Drawing for the job (mm, zero at the part's lowest x, y, z). A direction names the side the tool comes from. Give positions to 0.01 mm unless a question says otherwise; leave off trailing zeros. Loops run counter-clockwise (first coordinate to the right, second up) from the corner with the lowest first, then second, coordinate; pieces in that order, holes last. Notation, with made-up numbers: (89, 49) -> (96, 49) arc R17 cw to (96, 70) -> close; hole circle Ø9 at (65.5, -21.5). An arc over 180 degrees is marked (long way). Answer in a Markdown table with one row per item. Add a question column.
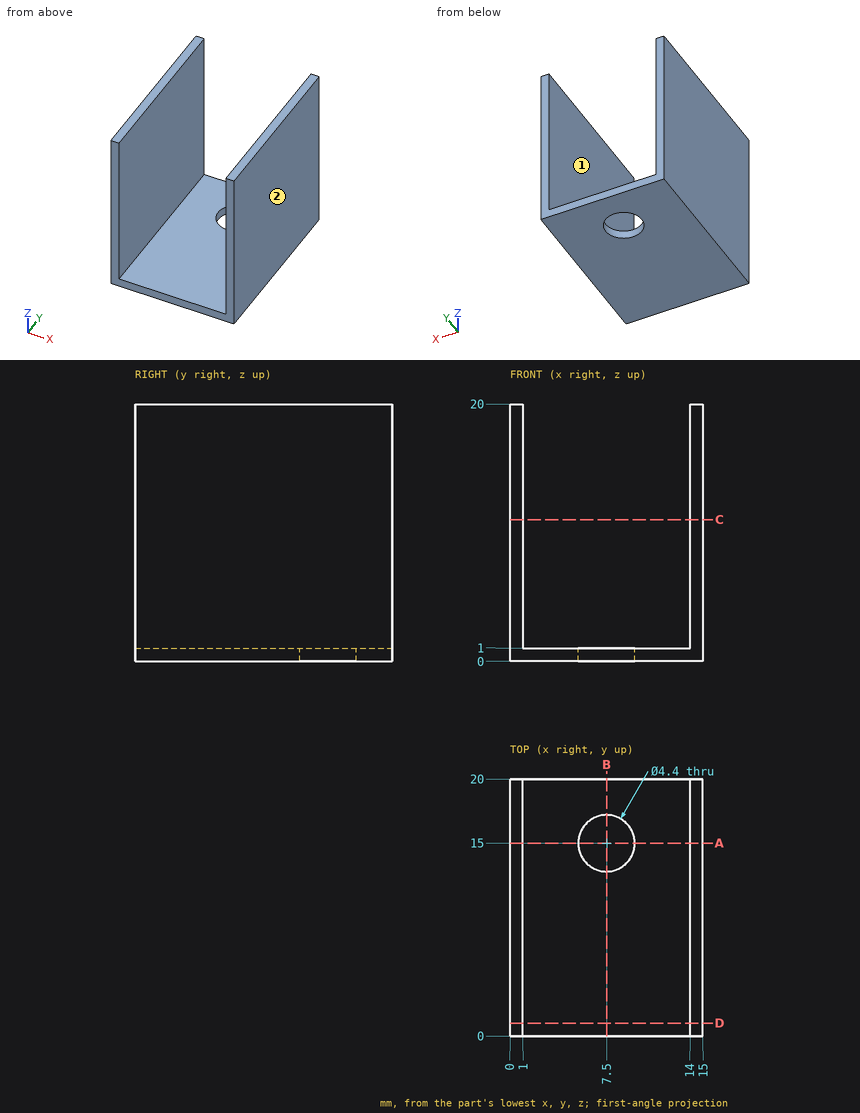
(1) Saw through at B-B, the plane x = 7.5. List the corners of the cut face in (y, z), then the cut area to 3 significant figures.
(2) Wall check: line 1 along X through (y, z) = (18, 8); line 2 along Y through (x, z) = (7.5, 0.7); line 3 along Z through (x, y) = (3.5, 11.5). Give the ranges that are in metal, low to high. Write a range as from..to.
(3) Saw through at D-D, the plane y = 1. List the corners of the cut face in (x, z).
(4) 3-axis set-ups, long thin cutter, end or side, ignore diameter. For the marked faces 1 and 2: which of +Z, -Z, +X, -X, +Y, -Y reach the whole face in a straight line?
(5) Saw through at C-C, the plane z = 11. List the corners of the cut face in (x, y), then the cut area to 3 significant figures.
(6) Saw through at A-A, the plane y = 15. List the corners of the cut face in (x, z), then the cut area to 3 significant figures.
(7) Flat gauge pin, fed straight in: pin 1 Ø3 at (x, y) = (4, 7.5) entering from +Z. Where does the tip first touch, or does it go through?
Worked answers:
| question | item | result |
|---|---|---|
| 1 | outline | (0, 0) -> (12.8, 0) -> (12.8, 1) -> (0, 1) -> close; (17.2, 0) -> (20, 0) -> (20, 1) -> (17.2, 1) -> close |
| 1 | area | 15.6 mm^2 |
| 2 | line 1 | 0..1, 14..15 |
| 2 | line 2 | 0..12.8, 17.2..20 |
| 2 | line 3 | 0..1 |
| 3 | outline | (0, 0) -> (15, 0) -> (15, 20) -> (14, 20) -> (14, 1) -> (1, 1) -> (1, 20) -> (0, 20) -> close |
| 4 | face 1 | +Z, +Y, -Y |
| 4 | face 2 | +Z, -Z, +X, +Y, -Y |
| 5 | outline | (0, 0) -> (1, 0) -> (1, 20) -> (0, 20) -> close; (14, 0) -> (15, 0) -> (15, 20) -> (14, 20) -> close |
| 5 | area | 40.0 mm^2 |
| 6 | outline | (0, 0) -> (5.3, 0) -> (5.3, 1) -> (1, 1) -> (1, 20) -> (0, 20) -> close; (9.7, 0) -> (15, 0) -> (15, 20) -> (14, 20) -> (14, 1) -> (9.7, 1) -> close |
| 6 | area | 48.6 mm^2 |
| 7 | pin 1 | z = 1 |
